Autodesk Inventor part; units mm, degrees
ref_plane "YZ Plane" through (0, 0, 0) normal (1, 0, 0) x (0, 1, 0)
ref_plane "XZ Plane" through (0, 0, 0) normal (0, 1, 0) x (-1, 0, 0)
ref_plane "XY Plane" through (0, 0, 0) normal (0, 0, 1) x (1, 0, 0)
sketch "Esboço2" plane through (0, 0, 0) normal (1, 0, 0) x (0, 1, 0)
  circle A0 centre (0, 0) radius 4.7625
  dimension "d0" = 9.525
extrude "Extrusão1" add sketch "Esboço2" along normal blind 6
sketch "Esboço3" plane through (6, 0, 0) normal (1, 0, 0) x (0, 0, -1)
  circle A0 centre (0, 0) radius 4.7625
  circle A1 centre (0, 0) radius 3.5719
  dimension "d3" = 7.1437
extrude "Extrusão2" add sketch "Esboço3" along normal blind 1 contours A1
sketch "Esboço4" plane through (7, 0, 0) normal (1, 0, 0) x (0, 0, -1)
  circle A0 centre (0, 0) radius 3.5719
  circle A1 centre (0, 0) radius 4.7625
  dimension "d6" = 9.525
extrude "Extrusão3" add sketch "Esboço4" along normal blind 50 contours A0 | A1
chamfer "Chanfro1" distance 0.5 angle 45 2 edges at (0, -4.7625, 0) (57, 0, 4.7625)
sketch "Esboço7" plane through (0, 0, 0) normal (0, 0, 1) x (1, 0, 0)
  line L0 (57, 4.2625) -> (57, -4.2625)
  line L1 (0, -4.2625) -> (0, 4.2625)
  point P0 (0, 0)
  point P1 (54, 0)
  point P2 (3, 0)
  dimension "d18" = 3
  dimension "d33" = 3
hole "Furo1" at (54, 0, 0) at (3, 0, 0) direction (0, 0, -1) diameter 3 end through all
hole "Furo2" at (54, 0, 0) at (3, 0, 0) direction (0, 0, 1) diameter 3 end through all
properties part number "pino_a3" material "Aço carbono"
The model under review builds one solid part; all positions refer to its coordinate system, in mm. A direction names the side the tool comes from. Coordinates: 2 decimals unless noted, no trailing zeros. Order: outer loops, then holes, each group sorted by start corner. A loop starts at its lowest first (then second) coordinate and runs counter-clockwise, first axis right, second up. Notation, with made-up numbers: (10.25, -39) -> (65.25, -39) arc R12 cw to (65.25, -25) -> close; hole circle Ø4 at (72.25, 41.25). An arc over 180 degrees is marked (long way). Answer in a Markdown table with one row per item. Add a question column.
Item 1: We need section D-D on x = 11.5. Write out the cut boundary in (y, z) (1 decimal).
Item 2: We need section B-B on y = 0. Write out the cut boundary in (x, z).
Item 3: Mouldability with a two-part tool opening along Y and no side actions: class faces 1 (the flat face through (0, 0, 0)), 2 (the cylindrical face through (52.503, -0.099, -0.067)), 3 (the cylindrical face through (3.212, 4.543, -1.431)) as +Y half, -Y half, draft (parallel to the pull), parting line (faces both ways), or undercut.
Item 4: To check wall thickness, follow probe 1 along X at (y, z) = (-0.25, 2.5); probe 2 along X at (y, z) = (4, 1.25); probe 3 along X at (y, z) = (-4, 2). State the ranges of each line that lie inside material, in increasing order.
Item 5: Machinability: for faces 4 (the cylindrical face through (1.503, -0.099, -0.067)), 5 (the flat face through (6, 1, 4)), which of the approach directions +Z, -Z, +X, -X, +Y, -Y give a long, thin tool a straight path to every point of the face, cutting with its end or side? Answer none if there is none.
Item 6: We need section C-C on x = 54. Write out the cut boundary in (y, z) (1 decimal), plus the area to 3 significant figures.
Item 7: We need section A-A on z = 0. Write out the cut boundary in (x, y), plus the area to 3 significant figures.
Final values:
| question | item | result |
|---|---|---|
| 1 | outline | circle Ø9.5 at (0, 0) |
| 2 | outline | (0, -4.26) -> (0.5, -4.76) -> (1.5, -4.76) -> (1.5, 4.76) -> (0.5, 4.76) -> (0, 4.26) -> close; (4.5, -4.76) -> (6, -4.76) -> (6, -3.57) -> (7, -3.57) -> (7, -4.76) -> (52.5, -4.76) -> (52.5, 4.76) -> (7, 4.76) -> (7, 3.57) -> (6, 3.57) -> (6, 4.76) -> (4.5, 4.76) -> close; (55.5, -4.76) -> (56.5, -4.76) -> (57, -4.26) -> (57, 4.26) -> (56.5, 4.76) -> (55.5, 4.76) -> close |
| 3 | face 1 | draft |
| 3 | face 2 | undercut |
| 3 | face 3 | parting line |
| 4 | probe 1 | x = 0 to 1.52, 4.48 to 52.52, 55.48 to 57 |
| 4 | probe 2 | x = 0 to 6, 7 to 57 |
| 4 | probe 3 | x = 0.21 to 6, 7 to 56.79 |
| 5 | face 4 | +Z, -Z |
| 5 | face 5 | none |
| 6 | outline | (-1.5, -4.5) -> (-1.5, 4.5) arc R4.8 ccw to start; (1.5, -4.5) arc R4.8 ccw to (1.5, 4.5) -> close |
| 6 | area | 43.2 mm2 |
| 7 | outline | (0, -4.26) -> (0.5, -4.76) -> (6, -4.76) -> (6, -3.57) -> (7, -3.57) -> (7, -4.76) -> (56.5, -4.76) -> (57, -4.26) -> (57, 4.26) -> (56.5, 4.76) -> (7, 4.76) -> (7, 3.57) -> (6, 3.57) -> (6, 4.76) -> (0.5, 4.76) -> (0, 4.26) -> close; hole circle Ø3 at (3, 0); hole circle Ø3 at (54, 0) |
| 7 | area | 526 mm2 |
